Answer from the drawing. Dimensions are ordinates in mm from the lowest x, y and z of the part. Give positions to 0.01 mm unless a question says otherwise; leave off trailing zeros. Order: outer loops, then holes, each group sorted by start corner. A loop starts at its lowest first (then second) coordinate and runs counter-clockwise, first axis right, second up. Notation, with made-up numbers: (-17.5, 11) -> (-11.5, 11) arc R15 cw to (-11.5, 38) -> close; hole circle Ø4 at (14, 74). An arc over 180 degrees is marked (long way). Answer as CSV lines item,"result". Start each with the question number.
1) Straight lines are drawn through the part: L1, parallel to Y at x = 120, z = 56; L2, parallel to X at y = 35, z = 54.5; L3, parallel to Z at x = 56, y = 9. For each, find the intervals that lie inside material, in ascending order. Write a range as from..to.
2) The mould has two halves that part along X. Classify the marked faces 1, 2 and 3: +X half, -X half, draft (parallel to the pull), parting line (faces both ways), or undercut.
3) Find section C-C (x = 20). Determine the outline of the cut face in (y, z).
4) Find section D-D (y = 50). Determine the outline of the cut face in (x, z), and give its area (3 significant figures).
5) Find section A-A (x = 120). Determine the outline of the cut face in (y, z).
6) Find section B-B (y = 30). Determine the outline of the cut face in (x, z).
7) Flat-ended cylindrical pins translate along their axes: pin 1 Ø10 at (x, y) = (123.5, 27.5) entering from +Z; pin 2 Ø2 at (x, y) = (92, 44.5) entering from +Z. Find the tip coordinate at first contact, or state that the pin passes through.
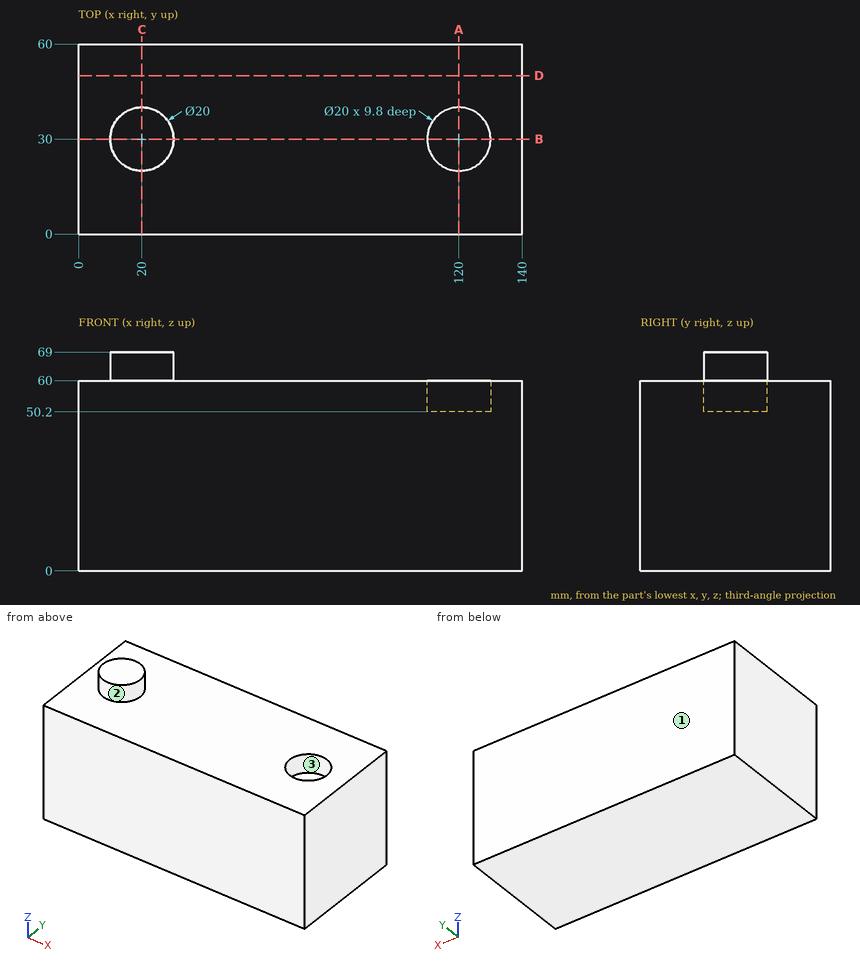
Findings below:
1,L1,"0..20, 40..60"
1,L2,"0..111.34, 128.66..140"
1,L3,"0..60"
2,face 1,"draft"
2,face 2,"parting line"
2,face 3,"undercut"
3,outline,"(0, 0) -> (60, 0) -> (60, 60) -> (40, 60) -> (40, 69) -> (20, 69) -> (20, 60) -> (0, 60) -> close"
4,outline,"(0, 0) -> (140, 0) -> (140, 60) -> (0, 60) -> close"
4,area,"8,400 mm²"
5,outline,"(0, 0) -> (60, 0) -> (60, 60) -> (40, 60) -> (40, 50.2) -> (20, 50.2) -> (20, 60) -> (0, 60) -> close"
6,outline,"(0, 0) -> (140, 0) -> (140, 60) -> (130, 60) -> (130, 50.2) -> (110, 50.2) -> (110, 60) -> (30, 60) -> (30, 69) -> (10, 69) -> (10, 60) -> (0, 60) -> close"
7,pin 1,"z = 50.2"
7,pin 2,"z = 60"
